CAD build for the part. Positions are in the model's coordinates, mm. A direction names the side the tool comes from. Round coordinates to 2 decimals unless told otherwise and drop trailing zeros. Write each loop counter-clockwise with the first axis right and the second up, starting at its lowest first coordinate (ties: lowest second). Pieces come first, ordered by that corner, then holes. Notation, with made-up numbers: (66, 22) - (125, 22) arc R12 cw to (125, 37) - close; hole circle Ø10 at (46, 76). An arc over 180 degrees is marked (long way). Put each result on its own line as item: value. Start each with the question number.
Item 1: Drill centre lines: line 1 (X direction, y = -1.2, z = 8.5); line 2 (Y direction, x = 0.95, z = 6.25); line 3 (Y direction, x = 0.1, z = 2.75). Where is each one in solid material? Low to high. Write a range as from..to.
Item 2: Cut at A-A (x = 0). Give the cut face in (y, z).
Item 3: Mould opens along Y. For faces 1 (the flat face through (0.5, -1, 10)), 2 (the flat face through (0.2, 1, 5)), 3 (the cylindrical face through (1.29, 2.024, 4.93)) say: released by +Y, released by -Y, zero draft, split by the parting line, or undercut.
Item 4: 3-axis set-ups, long thin cutter, end or side, ignore diameter. For faces 4 (the flat face through (-1, 0.2, 5)), 5 (the flat face through (0.5, -1, 0)): which of +Z, -Z, +X, -X, +Y, -Y reach the whole face in a straight line?
Item 5: Cut at D-D (y = 0.85). Give the cut face in (x, z).
Item 6: Pin check, flat tips, straight feed: pin 1 Ø1 at (x, z) = (1.5, 7.5) entering from -Y; pin 2 Ø1 at (y, z) = (-1.5, 3) entering from -X; pin 3 Ø0.6 at (y, z) = (1.5, 3.5) entering from +X. Stop position of each tip, or through.
```python
from build123d import *

# Parameters (mm, degrees)
F0_R     = 2.4
F1_DEPTH = 10


with BuildPart() as f1:
    # F0 (on Top) → F1 (new body)
    with BuildSketch(Plane.XY):
        Circle(F0_R)
        with BuildLine():
            ThreePointArc((-1.548546, 1.265703), (-1.414214, 1.414214), (-1.265703, 1.548546))
            Line((-1.265703, 1.548546), (-0.369705, 0.652548))
            ThreePointArc((-0.369705, 0.652548), (-0.287013, 0.69291), (-0.2, 0.722842))
            Line((-0.2, 0.722842), (-0.2, 1.989975))
            ThreePointArc((-0.2, 1.989975), (0, 2), (0.2, 1.989975))
            Line((0.2, 1.989975), (0.2, 0.722842))
            ThreePointArc((0.2, 0.722842), (0.287013, 0.69291), (0.369705, 0.652548))
            Line((0.369705, 0.652548), (1.265703, 1.548546))
            ThreePointArc((1.265703, 1.548546), (1.414214, 1.414214), (1.548546, 1.265703))
            Line((1.548546, 1.265703), (0.652548, 0.369705))
            ThreePointArc((0.652548, 0.369705), (0.69291, 0.287013), (0.722842, 0.2))
            Line((0.722842, 0.2), (1.989975, 0.2))
            ThreePointArc((1.989975, 0.2), (2, 0), (1.989975, -0.2))
            Line((1.989975, -0.2), (0.722842, -0.2))
            ThreePointArc((0.722842, -0.2), (0.69291, -0.287013), (0.652548, -0.369705))
            Line((0.652548, -0.369705), (1.548546, -1.265703))
            ThreePointArc((1.548546, -1.265703), (1.414214, -1.414214), (1.265703, -1.548546))
            Line((1.265703, -1.548546), (0.369705, -0.652548))
            ThreePointArc((0.369705, -0.652548), (0.287013, -0.69291), (0.2, -0.722842))
            Line((0.2, -0.722842), (0.2, -1.989975))
            ThreePointArc((0.2, -1.989975), (0, -2), (-0.2, -1.989975))
            Line((-0.2, -1.989975), (-0.2, -0.722842))
            ThreePointArc((-0.2, -0.722842), (-0.287013, -0.69291), (-0.369705, -0.652548))
            Line((-0.369705, -0.652548), (-1.265703, -1.548546))
            ThreePointArc((-1.265703, -1.548546), (-1.414214, -1.414214), (-1.548546, -1.265703))
            Line((-1.548546, -1.265703), (-0.652548, -0.369705))
            ThreePointArc((-0.652548, -0.369705), (-0.69291, -0.287013), (-0.722842, -0.2))
            Line((-0.722842, -0.2), (-1.989975, -0.2))
            ThreePointArc((-1.989975, -0.2), (-2, 0), (-1.989975, 0.2))
            Line((-1.989975, 0.2), (-0.722842, 0.2))
            ThreePointArc((-0.722842, 0.2), (-0.69291, 0.287013), (-0.652548, 0.369705))
            Line((-0.652548, 0.369705), (-1.548546, 1.265703))
        make_face(mode=Mode.SUBTRACT)
    extrude(amount=F1_DEPTH)


solid = f1.part
```
Output values:
1. line 1: -2.08..-1.48, -0.92..-0.2, 0.2..0.92, 1.48..2.08
1. line 2: -2.2..-1.23, -0.67..-0.2, 0.2..0.67, 1.23..2.2
1. line 3: -2.4..-2, 2..2.4
2. outline: (-2.4, 0) - (-2, 0) - (-2, 10) - (-2.4, 10) - close; (2, 0) - (2.4, 0) - (2.4, 10) - (2, 10) - close
3. face 1: zero draft
3. face 2: undercut
3. face 3: split by the parting line
4. face 4: +Z, -Z
4. face 5: -Z, +X, -X, +Y, -Y
5. outline: (-2.24, 0) - (-1.13, 0) - (-1.13, 10) - (-2.24, 10) - close; (-0.57, 0) - (-0.2, 0) - (-0.2, 10) - (-0.57, 10) - close; (0.2, 0) - (0.57, 0) - (0.57, 10) - (0.2, 10) - close; (1.13, 0) - (2.24, 0) - (2.24, 10) - (1.13, 10) - close
6. pin 1: y = -2.18
6. pin 2: x = -2.18
6. pin 3: x = 2.08
